```python
from build123d import *

# Parameters (mm, degrees)
SKETCH1_R           = 49.638488844
SKETCH1_R_2         = 46.667664218
BOSS_EXTRUDE1_DEPTH = 7.5
SKETCH2_W           = 16.879419562
SKETCH2_H           = 14.533093082
SKETCH2_W_2         = 10
SKETCH2_H_2         = 8
BOSS_EXTRUDE2_DEPTH = 15
FILLET1_R           = 4


with BuildPart() as part:
    # Sketch1 → Boss-Extrude1 (new, symmetric)
    with BuildSketch(Plane.XY):
        Circle(SKETCH1_R)
        Circle(SKETCH1_R_2, mode=Mode.SUBTRACT)
    extrude(amount=BOSS_EXTRUDE1_DEPTH, both=True)

    # Sketch2 → Boss-Extrude2 (add)
    with BuildSketch(Plane(origin=(0, 0, -7.5), x_dir=(-1, 0, 0), z_dir=(0, 0, -1))):
        with Locations((0, 55.024649482)):
            Rectangle(SKETCH2_W, SKETCH2_H)
        with Locations((0, 55.024649482)):
            Rectangle(SKETCH2_W_2, SKETCH2_H_2, mode=Mode.SUBTRACT)
    extrude(amount=-BOSS_EXTRUDE2_DEPTH)

    # Fillet1
    fillet1_edges = [part.edges().sort_by_distance(p)[0] for p in [
        (-8.439709781, 62.291196023, 0),
        (8.439709781, 62.291196023, 0),
    ]]
    fillet(fillet1_edges, radius=FILLET1_R)


solid = part.part
```
Check sheet for the modelled part. Datum: model origin and axes. Units: mm. A direction names the side the tool comes from. Coordinates: 2 decimals unless noted, no trailing zeros. Order: outer loops, then holes, each group sorted by start corner. A loop starts at its lowest first (then second) coordinate and runs counter-clockwise, first axis right, second up. Notation, with made-up numbers: (8, -6) -> (64, -6) arc R21 cw to (64, 26) -> close; hole circle Ø10 at (-12, 16). An arc over 180 degrees is marked (long way). Write item = value, one per line. Start each with the question number.
1) Cross-section at B-B (x = 0). Enter the section's corners in (y, z).
2) Cross-section at C-C (x = 33.5). Enter the section's corners in (y, z).
3) Cross-section at D-D (z = -0.75). Enter the section's corners in (x, y), then the cut area to 3 significant figures.
4) Mould release check, pull along X, two halves, no side actions. Record for faces 1 (the flat face through (0, 59.025, 0)), 2 (the flat face through (0, 62.291, 0)), 3 (the flat face through (-8.44, 54, 0)): +X half, -X half, draft (parallel to the pull), parting line (faces both ways), or undercut.
5) Access from +Z, -Z, +X, -X, +Y, -Y to the whole of each face (thin tool, end or side, straight path). Record for faces 4 (the flat face through (8.44, 54, 0)), 5 (the flat face through (5, 55, 0)), 6 (the flat face through (0, 48, 7.5)).
6) Material ranges on L1, parallel to Y at x = 0, z = -4; L2, parallel to X at y = -37, z = 6.25; L3, parallel to X at y = 16.5, z = -2.25, recorded low to high.
7) Cross-section at A-A (y = 0). Enter the section's corners in (x, z), then the cut area to 3 significant figures.
8) Go/stop test with flat-tipped pins: P1, Ø5, axis at x = -1.5, z = 2, coming from the -Y side; P2, Ø8, axis at x = -15.5, z = 5, coming from the +Y side; P3, Ø6.5, axis at y = 56.5, z = -2.5, coming from the +X side. Record where each tip stops, or that it passes through.
Ans:
q1.outline = (-49.64, -7.5) -> (-46.67, -7.5) -> (-46.67, 7.5) -> (-49.64, 7.5) -> close; (46.67, -7.5) -> (51.02, -7.5) -> (51.02, 7.5) -> (46.67, 7.5) -> close; (59.02, -7.5) -> (62.29, -7.5) -> (62.29, 7.5) -> (59.02, 7.5) -> close
q2.outline = (-36.63, -7.5) -> (-32.49, -7.5) -> (-32.49, 7.5) -> (-36.63, 7.5) -> close; (32.49, -7.5) -> (36.63, -7.5) -> (36.63, 7.5) -> (32.49, 7.5) -> close
q3.outline = (-8.44, 48.92) arc R49.64 ccw (long way) to (8.44, 48.92) -> (8.44, 58.29) arc R4 ccw to (4.44, 62.29) -> (-4.44, 62.29) arc R4 ccw to (-8.44, 58.29) -> close; hole circle Ø93.34 at (0, 0); hole (-5, 51.02) -> (5, 51.02) -> (5, 59.02) -> (-5, 59.02) -> close
q3.area = 1,030 mm²
q4.face_1 = undercut
q4.face_2 = draft
q4.face_3 = -X half
q5.face_4 = +Z, -Z, +X, +Y
q5.face_5 = +Z, -Z
q5.face_6 = +Z, +X, -X, +Y, -Y
q6.L1 = -49.64 to -46.67, 46.67 to 51.02, 59.02 to 62.29
q6.L2 = -33.09 to -28.44, 28.44 to 33.09
q6.L3 = -46.82 to -43.65, 43.65 to 46.82
q7.outline = (-49.64, -7.5) -> (-46.67, -7.5) -> (-46.67, 7.5) -> (-49.64, 7.5) -> close; (46.67, -7.5) -> (49.64, -7.5) -> (49.64, 7.5) -> (46.67, 7.5) -> close
q7.area = 89.1 mm²
q8.P1 = -49.64
q8.P2 = 48.29
q8.P3 = 8.44
